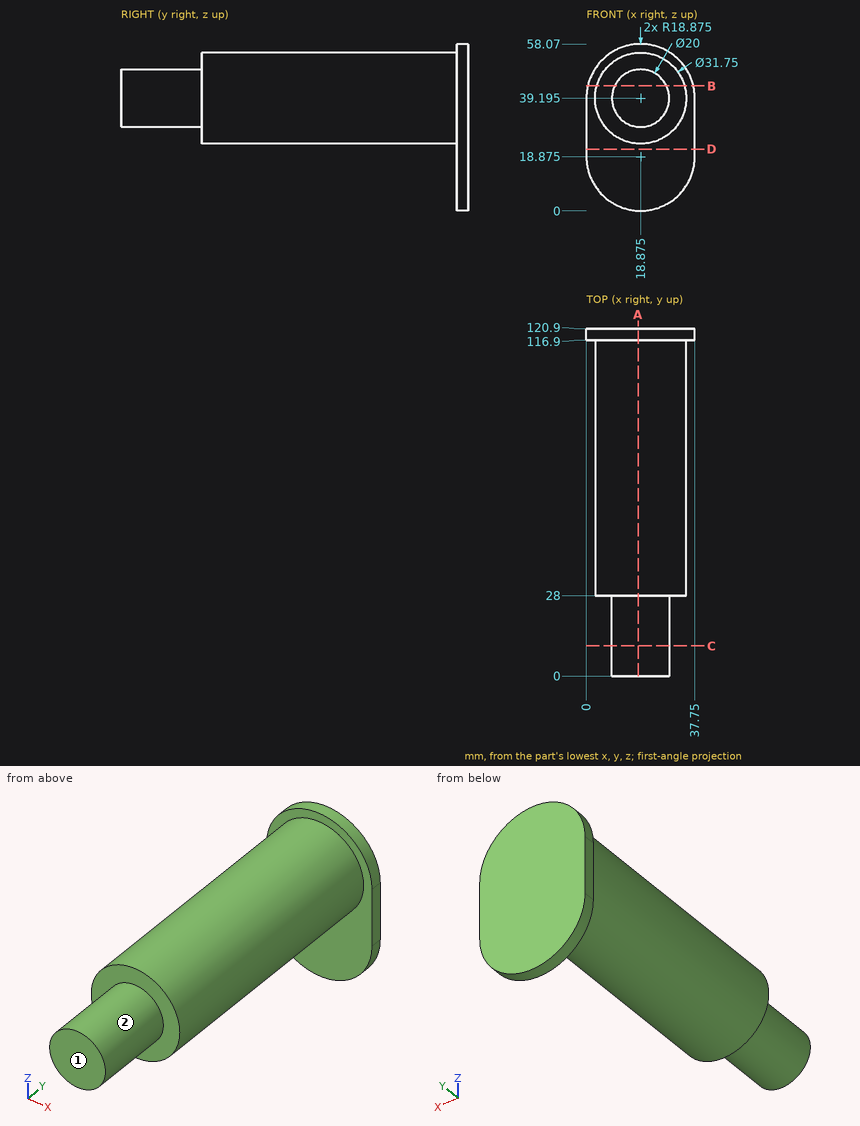
For this review, use the dimensioned drawing (mm, ordinates from the lowest corner) and the shaded views. A direction names the side the tool comes from. Round coordinates to 2 decimals unless told otherwise and drop trailing zeros. Write each loop counter-clockwise with the first axis right and the second up, starting at its lowest first coordinate (ties: lowest second). Pieces come first, ordered by that corner, then holes. Notation, with made-up numbers: M -22.75,11.25 L -16.75,11.25 A29 ccw -16.75,34.25 Z; hole C 87.25,-21 d11. An arc over 180 degrees is marked long. Use CSV: the item, a comma, the result in double quotes. Start each with the question number.
(1) Clearance check with flat-ended pins moving along their axes: P1, Ø12, axis at y = 65, z = 47, coming from the +X side; P2, Ø8, axis at y = 82.5, z = 22, coming from the -X side; P3, Ø6, axis at y = 50, z = 32.5, coming from the -X side. State where each tip first meets the part, or that it passes through.
(2) We need section B-B, the plane z = 43.5. State the section outline as (x, y) points.
(3) We need section D-D, the plane z = 21.5. State the section outline as (x, y) points, then the cut area to 3 significant figures.
(4) Tool access review of the marked faces 1 and 2: name each direction out of +Z, -Z, +X, -X, +Y, -Y from which nothing blocks a thin tool from reaching the whole face with its end or side.
(5) We need section C-C, the plane y = 10.5. State the section outline as (x, z) points (3 decimals), then the cut area to 3 significant figures.
(6) We need section A-A, the plane x = 18. State the section outline as (y, z) points.
(7) For line 1 along Y through (x, z) = (8.5, 30); line 2 along Y through (x, z) = (34.5, 49.5); line 3 along X through (y, z) = (63.5, 51.5), list the stretches that pass through material, from the lowest coordinate up.
Findings:
1,P1,"x = 34.65"
1,P2,"x = 10.05"
1,P3,"x = 3.44"
2,outline,"M 0.5,116.9 L 3.59,116.9 L 3.59,28 L 9.85,28 L 9.85,0 L 27.9,0 L 27.9,28 L 34.16,28 L 34.16,116.9 L 37.25,116.9 L 37.25,120.9 L 0.5,120.9 Z"
3,outline,"M 0,116.9 L 37.75,116.9 L 37.75,120.9 L 0,120.9 Z"
3,area,"151 mm^2"
4,face 1,"+Z, -Z, +X, -X, -Y"
4,face 2,"-Y"
5,outline,"C 18.875,39.195 d20"
5,area,"314 mm^2"
6,outline,"M 0,29.23 L 28,29.23 L 28,23.34 L 116.9,23.34 L 116.9,0.02 L 120.9,0.02 L 120.9,58.05 L 116.9,58.05 L 116.9,55.05 L 28,55.05 L 28,49.16 L 0,49.16 Z"
7,line 1,"28 to 120.9"
7,line 2,"116.9 to 120.9"
7,line 3,"8.84 to 28.91"
